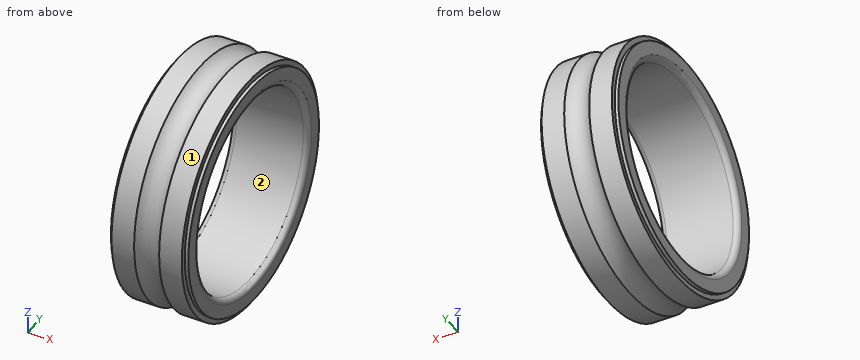
Autodesk Inventor part; units mm, degrees
ref_plane "ip_cst_3_ir_1_1_XY" through (7, 24.25, 0) normal (-1, 0, 0) x (0, 0, -1)
ref_plane "ip_cst_3_ir_1_1_YZ" through (7, 24.25, 0) normal (0, 0, -1) x (0, -1, 0)
ref_plane "ip_cst_3_ir_1_1_ZX" through (7, 24.25, 0) normal (0, -1, 0) x (-1, 0, 0)
sketch "Sketch_1" plane through (0, 0, 0) normal (0, 0, 1) x (1, 0, 0)
  line L0 (14, 0) -> (0, 0)
  arc A0 (0, 18.5) -> (1, 17.5) centre (1, 18.5) ccw
  line L1 (1, 17.5) -> (13, 17.5)
  arc A1 (13, 17.5) -> (14, 18.5) centre (13, 18.5) ccw
  line L2 (14, 18.5) -> (14, 20.8)
  line L3 (14, 20.8) -> (13.356, 20.8)
  line L4 (13.356, 20.8) -> (13.356, 21.75)
  line L5 (13.356, 21.75) -> (9.2673, 21.75)
  arc A2 (4.7327, 21.75) -> (9.2673, 21.75) centre (7, 24.25) ccw
  line L6 (4.7327, 21.75) -> (0.644, 21.75)
  line L7 (0.644, 21.75) -> (0.644, 20.8)
  line L8 (0.644, 20.8) -> (0, 20.8)
  line L9 (0, 20.8) -> (0, 18.5)
revolve "Revolution1" add sketch "Sketch_1" angle 360 about axis through (14, 0, 0) along (1, 0, 0)
ref_plane "ip_cst_3_ir_1_1_XY" through (7, 24.25, 0) normal (-1, 0, 0) x (0, 0, -1)
ref_plane "ip_cst_3_ir_1_1_YZ" through (7, 24.25, 0) normal (0, 0, -1) x (0, -1, 0)
ref_plane "ip_cst_3_ir_1_1_ZX" through (7, 24.25, 0) normal (0, -1, 0) x (-1, 0, 0)
ref_plane "ip_cst_3_ir_1_10_XY" through (7, -8.5992, -22.6741) normal (-1, 0, 0) x (0, 0, -1)
ref_plane "ip_cst_3_ir_1_10_YZ" through (7, -8.5992, -22.6741) normal (0, 0, -1) x (0, -1, 0)
ref_plane "ip_cst_3_ir_1_10_ZX" through (7, -8.5992, -22.6741) normal (0, -1, 0) x (-1, 0, 0)
ref_plane "ip_cst_3_ir_1_11_XY" through (7, 2.923, -24.0732) normal (-1, 0, 0) x (0, 0, -1)
ref_plane "ip_cst_3_ir_1_11_YZ" through (7, 2.923, -24.0732) normal (0, 0, -1) x (0, -1, 0)
ref_plane "ip_cst_3_ir_1_11_ZX" through (7, 2.923, -24.0732) normal (0, -1, 0) x (-1, 0, 0)
ref_plane "ip_cst_3_ir_1_12_XY" through (7, 13.7756, -19.9574) normal (-1, 0, 0) x (0, 0, -1)
ref_plane "ip_cst_3_ir_1_12_YZ" through (7, 13.7756, -19.9574) normal (0, 0, -1) x (0, -1, 0)
ref_plane "ip_cst_3_ir_1_12_ZX" through (7, 13.7756, -19.9574) normal (0, -1, 0) x (-1, 0, 0)
ref_plane "ip_cst_3_ir_1_13_XY" through (7, 21.4723, -11.2695) normal (-1, 0, 0) x (0, 0, -1)
ref_plane "ip_cst_3_ir_1_13_YZ" through (7, 21.4723, -11.2695) normal (0, 0, -1) x (0, -1, 0)
ref_plane "ip_cst_3_ir_1_13_ZX" through (7, 21.4723, -11.2695) normal (0, -1, 0) x (-1, 0, 0)
ref_plane "ip_cst_3_ir_1_2_XY" through (7, 21.4723, 11.2695) normal (-1, 0, 0) x (0, 0, -1)
ref_plane "ip_cst_3_ir_1_2_YZ" through (7, 21.4723, 11.2695) normal (0, 0, -1) x (0, -1, 0)
ref_plane "ip_cst_3_ir_1_2_ZX" through (7, 21.4723, 11.2695) normal (0, -1, 0) x (-1, 0, 0)
ref_plane "ip_cst_3_ir_1_3_XY" through (7, 13.7756, 19.9574) normal (-1, 0, 0) x (0, 0, -1)
ref_plane "ip_cst_3_ir_1_3_YZ" through (7, 13.7756, 19.9574) normal (0, 0, -1) x (0, -1, 0)
ref_plane "ip_cst_3_ir_1_3_ZX" through (7, 13.7756, 19.9574) normal (0, -1, 0) x (-1, 0, 0)
ref_plane "ip_cst_3_ir_1_4_XY" through (7, 2.923, 24.0732) normal (-1, 0, 0) x (0, 0, -1)
ref_plane "ip_cst_3_ir_1_4_YZ" through (7, 2.923, 24.0732) normal (0, 0, -1) x (0, -1, 0)
ref_plane "ip_cst_3_ir_1_4_ZX" through (7, 2.923, 24.0732) normal (0, -1, 0) x (-1, 0, 0)
ref_plane "ip_cst_3_ir_1_5_XY" through (7, -8.5992, 22.6741) normal (-1, 0, 0) x (0, 0, -1)
ref_plane "ip_cst_3_ir_1_5_YZ" through (7, -8.5992, 22.6741) normal (0, 0, -1) x (0, -1, 0)
ref_plane "ip_cst_3_ir_1_5_ZX" through (7, -8.5992, 22.6741) normal (0, -1, 0) x (-1, 0, 0)
ref_plane "ip_cst_3_ir_1_6_XY" through (7, -18.1514, 16.0807) normal (-1, 0, 0) x (0, 0, -1)
ref_plane "ip_cst_3_ir_1_6_YZ" through (7, -18.1514, 16.0807) normal (0, 0, -1) x (0, -1, 0)
ref_plane "ip_cst_3_ir_1_6_ZX" through (7, -18.1514, 16.0807) normal (0, -1, 0) x (-1, 0, 0)
ref_plane "ip_cst_3_ir_1_7_XY" through (7, -23.5453, 5.8034) normal (-1, 0, 0) x (0, 0, -1)
ref_plane "ip_cst_3_ir_1_7_YZ" through (7, -23.5453, 5.8034) normal (0, 0, -1) x (0, -1, 0)
ref_plane "ip_cst_3_ir_1_7_ZX" through (7, -23.5453, 5.8034) normal (0, -1, 0) x (-1, 0, 0)
ref_plane "ip_cst_3_ir_1_8_XY" through (7, -23.5453, -5.8034) normal (-1, 0, 0) x (0, 0, -1)
ref_plane "ip_cst_3_ir_1_8_YZ" through (7, -23.5453, -5.8034) normal (0, 0, -1) x (0, -1, 0)
ref_plane "ip_cst_3_ir_1_8_ZX" through (7, -23.5453, -5.8034) normal (0, -1, 0) x (-1, 0, 0)
ref_plane "ip_cst_3_ir_1_9_XY" through (7, -18.1514, -16.0807) normal (-1, 0, 0) x (0, 0, -1)
ref_plane "ip_cst_3_ir_1_9_YZ" through (7, -18.1514, -16.0807) normal (0, 0, -1) x (0, -1, 0)
ref_plane "ip_cst_3_ir_1_9_ZX" through (7, -18.1514, -16.0807) normal (0, -1, 0) x (-1, 0, 0)
ref_plane "ip_cst_3_ir_1a_XY" through (0, 0, 0) normal (1, 0, 0) x (0, 0, -1)
ref_plane "ip_cst_3_ir_1a_YZ" through (0, 0, 0) normal (0, 0, -1) x (0, 1, 0)
ref_plane "ip_cst_3_ir_1a_ZX" through (0, 0, 0) normal (0, 1, 0) x (1, 0, 0)
properties part number "6007DDU Inner ring"
Work out the finished part from the listing and answer in its coordinate system (mm). Face numbers are marked on the shaded views. Round coordinates to 2 decimals unless told otherwise and drop trailing zeros. Write each loop counter-clockwise with the first axis right and the second up, starting at its lowest first coordinate (ties: lowest second). Pieces come first, ordered by that corner, then holes. Notation, with made-up numbers: (45, 60) - (96, 60) arc R14 cw to (96, 75) - close; hole circle Ø6 at (53.25, 52.25). An arc over 180 degrees is marked (long way). Return JSON: item names as keys, results as strings. Group by question number.
Q1. Find the intervals of material crossed by L1, parallel to Z at x = 10.25, y = 0; L2, parallel to Z at x = 7.5, y = -4.5; L3, parallel to X at y = -12, z = -18, in increasing order.
Q2. Each of these flat-tipped pins is pushed along its axis until it touches: pin 1 Ø4 at (x, z) = (11.5, -15.5) entering from -Y; pin 2 Ø2 at (x, z) = (5.5, 4.5) entering from -Y (3 decimals); pin 3 Ø1.5 at (x, z) = (6, 1.5) entering from +Y. Where does it stop, or does it pass through?
Q3. The part is cut by section A-A on y = 0. Write down the section's boundary in (x, z) (3 decimals).
Q4. The mould has two halves that part along Z. Classify the marked faces 1 and 2: released by +Z, released by -Z, zero draft, split by the parting line, or undercut.
Q5. The part is cut by section C-C on x = 10.75. Write down the section's boundary in (y, z), then the cut area to 3 significant figures.
Solved:
{
 "1": {"L1": "-21.75 to -17.5, 17.5 to 21.75", "L2": "-20.42 to -16.91, 16.91 to 20.42", "L3": "0.64 to 4.87, 9.13 to 13.36"},
 "2": {"pin 1": "y = -17.05", "pin 2": "y = -21.405", "pin 3": "y = 21.31"},
 "3": {"outline": "(0, -20.8) - (0.644, -20.8) - (0.644, -21.75) - (4.733, -21.75) arc R3.375 cw to (9.267, -21.75) - (13.356, -21.75) - (13.356, -20.8) - (14, -20.8) - (14, -18.5) arc R1 ccw to (13, -17.5) - (1, -17.5) arc R1 ccw to (0, -18.5) - close; (0, 18.5) arc R1 ccw to (1, 17.5) - (13, 17.5) arc R1 ccw to (14, 18.5) - (14, 20.8) - (13.356, 20.8) - (13.356, 21.75) - (9.267, 21.75) arc R3.375 cw to (4.733, 21.75) - (0.644, 21.75) - (0.644, 20.8) - (0, 20.8) - close"},
 "4": {"face 1": "split by the parting line", "face 2": "undercut"},
 "5": {"outline": "circle Ø43.5 at (0, 0); hole circle Ø35 at (0, 0)", "area": "524 mm²"}
}
